from build123d import *

# Parameters (mm, degrees)
SKETCH_1_R          = 127
EXTRUDE_1_DEPTH     = 100
FILLET_1_R          = 10
SKETCH_2_R          = 64.5
CUT_EXTRUDE_1_DEPTH = 39
FILLET_2_R          = 10


with BuildPart() as part:
    # 草图1 → 凸台-拉伸1 (new body)
    with BuildSketch(Plane(origin=(0, 0, 0), x_dir=(1, 0, 0), z_dir=(0, 1, 0))):
        with Locations(Location((0, 0, 0), (0, 0, 270))):
            Circle(SKETCH_1_R)
    extrude(amount=EXTRUDE_1_DEPTH)

    # 圆角1
    fillet_1_edges = [part.edges().sort_by_distance(p)[0] for p in [
        (0, 0, -127),
        (0, 100, -127),
    ]]
    fillet(fillet_1_edges, radius=FILLET_1_R)

    # 草图2 → 切除-拉伸1 (cut)
    with BuildSketch(Plane.XZ):
        with Locations(Location((0, 0, 0), (0, 0, 270))):
            Circle(SKETCH_2_R)
    extrude(amount=-CUT_EXTRUDE_1_DEPTH, mode=Mode.SUBTRACT)

    # 圆角2
    fillet_2_edges = [part.edges().sort_by_distance(p)[0] for p in [
        (0, 0, 64.5),
    ]]
    fillet(fillet_2_edges, radius=FILLET_2_R)


solid = part.part
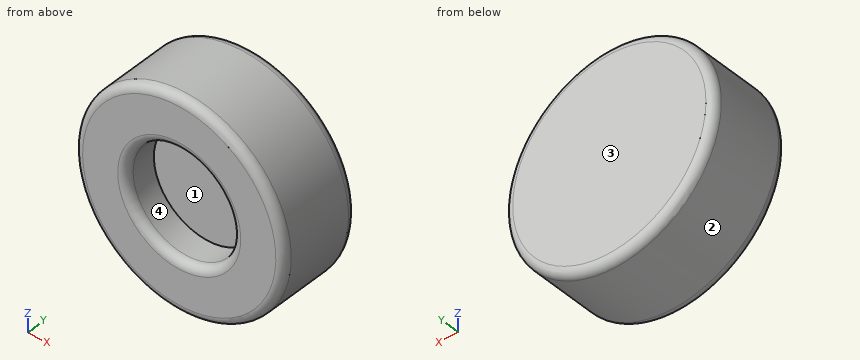
The listing builds one solid part. Answer for the finished solid, in the listing's coordinates (mm). Face numbers are marked on the shaded views. Give positions to 0.01 mm unless a question says otherwise; leave off trailing zeros. Write each loop counter-clockwise with the first axis right and the second up, starting at its lowest first coordinate (ties: lowest second). Pieces come first, ordered by that corner, then holes.
Item 1: Flat-ended cylindrical pins translate along their axes: P1, Ø5, axis at x = -58.5, z = -16.5, coming from the -Y side; P2, Ø1.5, axis at x = -7, z = -64.5, coming from the -Y side; P3, Ø6, axis at y = 55, z = -35, coming from the -X side. Find the tip coordinate at first contact, or state that the pin passes through.
Item 2: Find the intervals of material crossed by line 1 along X through (y, z) = (16, 0); line 2 along Y through (x, z) = (-39, -0.5); line 3 along X through (y, z) = (23, -13), in increasing order.
Item 3: Section B-B, the plane x = 0 is taken. Write down the section's boundary in (y, z).
Item 4: Section C-C, the plane y = 34 is taken. Write down the section's boundary in (x, z), plus the area to 3 significant figures.
Item 5: Determine the mould class of the marked faces 1, 2, 3 and 4 for opening direction Z: released by +Z, released by -Z, zero draft, split by the parting line, or undercut.
Item 6: Section A-A, the plane z = 0 is taken. Write down the section's boundary in (x, y).
Completed:
1. P1: stops at y = 39
1. P2: stops at y = 5.38
1. P3: stops at x = -122.9
2. line 1: x = -127 to -64.5, 64.5 to 127
2. line 2: y = 39 to 100
2. line 3: x = -126.33 to -63.18, 63.18 to 126.33
3. outline: (0, -117) arc R10 ccw to (10, -127) - (90, -127) arc R10 ccw to (100, -117) - (100, 117) arc R10 ccw to (90, 127) - (10, 127) arc R10 ccw to (0, 117) - (0, 74.5) arc R10 ccw to (10, 64.5) - (39, 64.5) - (39, -64.5) - (10, -64.5) arc R10 ccw to (0, -74.5) - close
4. outline: circle Ø254 at (0, 0); hole circle Ø129 at (0, 0)
4. area: 37,600 mm2
5. face 1: undercut
5. face 2: split by the parting line
5. face 3: zero draft
5. face 4: undercut
6. outline: (-127, 10) arc R10 ccw to (-117, 0) - (-74.5, 0) arc R10 ccw to (-64.5, 10) - (-64.5, 39) - (64.5, 39) - (64.5, 10) arc R10 ccw to (74.5, 0) - (117, 0) arc R10 ccw to (127, 10) - (127, 90) arc R10 ccw to (117, 100) - (-117, 100) arc R10 ccw to (-127, 90) - close
